```python
from build123d import *

# Parameters (mm, degrees)
EXTRUDE_1_DEPTH     = 1000
CUT_EXTRUDE_1_DEPTH = 1001.177984161
CUT_EXTRUDE_2_DEPTH = 1001.177984161


with BuildPart() as part:
    # Эскиз1 → Бобышка-Вытянуть1 (new body)
    with BuildSketch(Plane.XY):
        Polygon((-10, 0), (10, 0), (10, 4), (-6, 4), (-6, 20), (-10, 20), align=None)
    extrude(amount=EXTRUDE_1_DEPTH)

    # Эскиз2 → Вырез-Вытянуть1 (cut, through all)
    with BuildSketch(Plane(origin=(0, 4, 0), x_dir=(1, 0, 0), z_dir=(0, 1, 0))):
        Polygon((-6, 0), (10, -16), (10, 0), align=None)
    extrude(amount=-CUT_EXTRUDE_1_DEPTH, mode=Mode.SUBTRACT)

    # Эскиз3 → Вырез-Вытянуть2 (cut, through all)
    with BuildSketch(Plane(origin=(0, 4, 0), x_dir=(1, 0, 0), z_dir=(0, 1, 0))):
        Polygon((-6, -1000), (10, -984), (10, -1000), align=None)
    extrude(amount=-CUT_EXTRUDE_2_DEPTH, mode=Mode.SUBTRACT)


solid = part.part
```
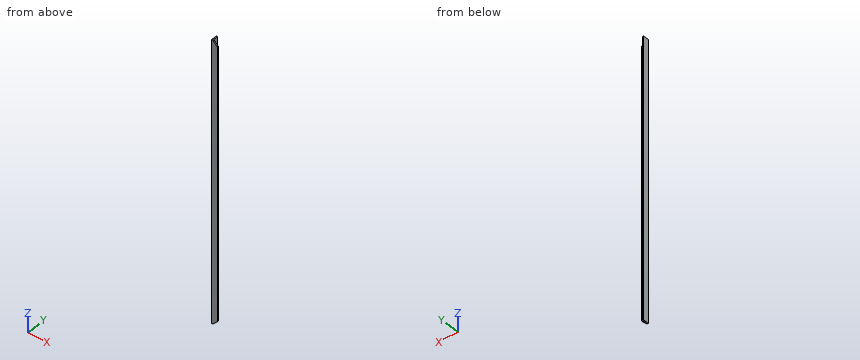
Work out the finished part from the listing and answer in its coordinate system (mm). Give positions to 0.01 mm unless a question says otherwise; leave off trailing zeros. Order: outer loops, then holes, each group sorted by start corner. A loop starts at its lowest first (then second) coordinate and runs counter-clockwise, first axis right, second up. Notation, with made-up numbers: (77, 62) -> (136, 62) arc R18 cw to (136, 88) -> close; hole circle Ø10 at (19.25, -24). An arc over 180 degrees is marked (long way). Answer as CSV lines item,"result". Start each with the question number.
(1) Section B-B, the plane x = 6.25 is taken. Write down the section's boundary in (y, z), plus the area to 3 significant figures.
(2) Section A-A, the plane z = 879 is taken. Write down the section's boundary in (x, y), plus the area to 3 significant figures.
(3) Consider line 1 along X through (y, z) = (4.5, 868.5); line 2 along Y through (x, z) = (-5.5, 488); line 3 along Z through (x, y) = (2.5, 3.75). Determine where each line is inside the solid, lowest interval first.
(4) Section C-C, the plane y = 8.75 is taken. Write down the section's boundary in (x, z), plus the area to 3 significant figures.
(5) Each of these flat-tipped pins is pushed along its axis until it touches: pin 1 Ø8 at (y, z) = (15.5, 381.5) entering from +X; pin 2 Ø8 at (x, z) = (2.5, 290) entering from +Y; pin 3 Ø1 at (x, y) = (-3, 3) entering from +Z. Where does it stop, or does it pass through?
Entries:
1,outline,"(0, 12.25) -> (4, 12.25) -> (4, 987.75) -> (0, 987.75) -> close"
1,area,"3,900 mm²"
2,outline,"(-10, 0) -> (10, 0) -> (10, 4) -> (-6, 4) -> (-6, 20) -> (-10, 20) -> close"
2,area,"144 mm²"
3,line 1,"-10 to -6"
3,line 2,"0 to 4"
3,line 3,"8.5 to 991.5"
4,outline,"(-10, 0) -> (-6, 0) -> (-6, 1000) -> (-10, 1000) -> close"
4,area,"4,000 mm²"
5,pin 1,"x = -6"
5,pin 2,"y = 4"
5,pin 3,"z = 997.5"
